Drawing for the job (mm, zero at the part's lowest x, y, z). Coordinates: 2 decimals unless noted, no trailing zeros. Order: outer loops, then holes, each group sorted by start corner. A loop starts at its lowest first (then second) coordinate and runs counter-clockwise, first axis right, second up. Notation, with made-up numbers: (31, 55) -> (57, 55) arc R17 ccw to (57, 62) -> close; hole circle Ø11 at (78.5, 36.5). An arc over 180 degrees is marked (long way). Write each question's results on one line, items separated by ' | '.
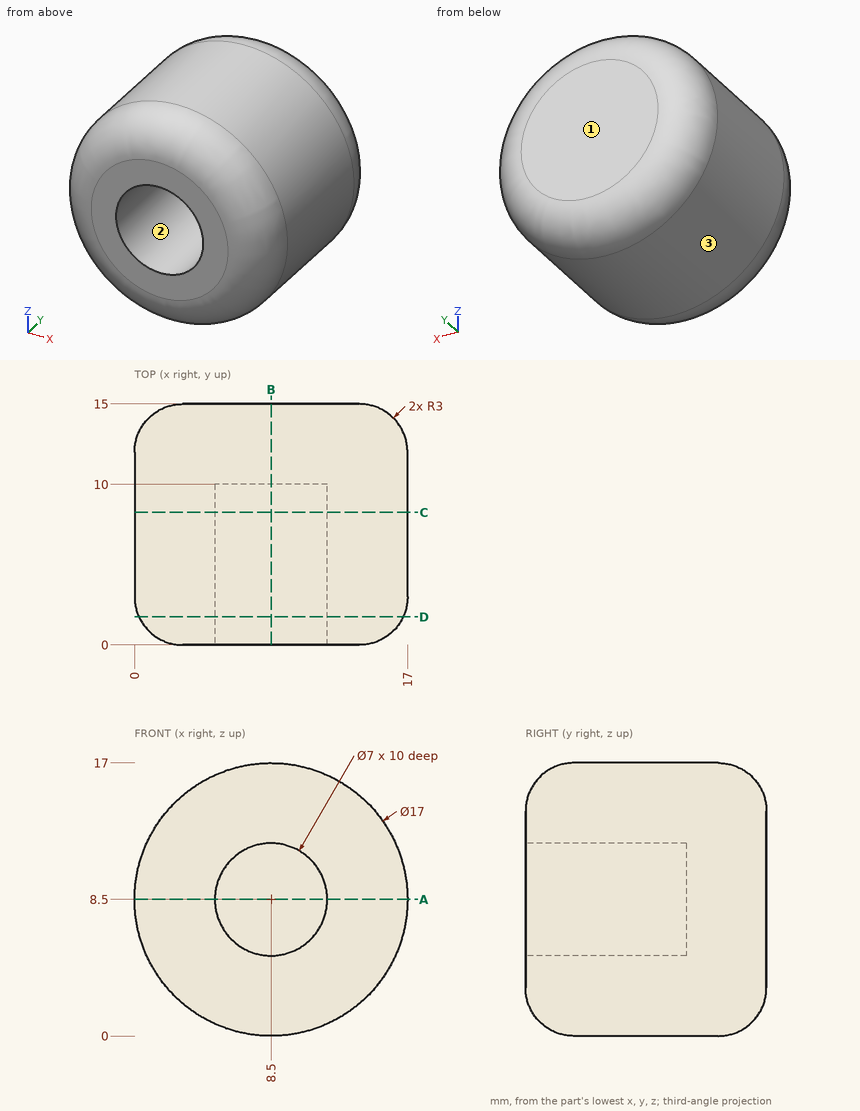
Item 1: Pin check, flat tips, straight feed: pin 1 (6.5 mm diameter, centred on x = 8.5, z = 8.5, fed in from -Y); pin 2 (1 mm diameter, centred on x = 4, y = 7.5, fed in from +Z). Stop position of each tip, or through.
Answer:
pin 1: stops at y = 10 | pin 2: stops at z = 16
Item 2: Slice it at B-B, the plane x = 8.5. List the corners of the cut face in (y, z).
Answer:
outline: (0, 3) arc R3 ccw to (3, 0) -> (12, 0) arc R3 ccw to (15, 3) -> (15, 14) arc R3 ccw to (12, 17) -> (3, 17) arc R3 ccw to (0, 14) -> (0, 12) -> (10, 12) -> (10, 5) -> (0, 5) -> close
Item 3: Slice it at C-C, the plane y = 8.25. List the corners of the cut face in (x, z), and give its area (3 significant figures).
Answer:
outline: circle Ø17 at (8.5, 8.5); hole circle Ø7 at (8.5, 8.5) | area: 188 mm^2
Item 4: Pull direction X, two halves, no side cores. Call the marked faces 1, 2 and 3: released by +X, released by -X, zero draft, split by the parting line, or undercut.
Answer:
face 1: zero draft | face 2: undercut | face 3: split by the parting line
Item 5: Slice it at D-D, the plane y = 1.75. List the corners of the cut face in (x, z).
Answer:
outline: circle Ø16.45 at (8.5, 8.5); hole circle Ø7 at (8.5, 8.5)
Item 6: Drill centre lines: line 1 (Y direction, x = 9.75, z = 10.5); line 2 (Z direction, x = 8.5, y = 4); line 3 (Z direction, x = 9.5, y = 4). Where is each one in solid material? Low to high. Write a range as from..to.
Answer:
line 1: y = 10..15 | line 2: z = 0..5, 12..17 | line 3: z = 0.06..5.15, 11.85..16.94
Item 7: Slice it at A-A, the plane z = 8.5. List the corners of the cut face in (x, y).
Answer:
outline: (0, 3) arc R3 ccw to (3, 0) -> (5, 0) -> (5, 10) -> (12, 10) -> (12, 0) -> (14, 0) arc R3 ccw to (17, 3) -> (17, 12) arc R3 ccw to (14, 15) -> (3, 15) arc R3 ccw to (0, 12) -> close
